```python
from build123d import *

# Parameters (mm, degrees)
F0_W     = 23
F0_H     = 95
F1_DEPTH = 9
F2_W     = 5
F2_H     = 95
F3_DEPTH = 5
F4_R     = 2
F5_DEPTH = 12.446


with BuildPart() as f1:
    # F0 (on Top) → F1 (new body)
    with BuildSketch(Plane.XY):
        Rectangle(F0_W, F0_H)
    extrude(amount=F1_DEPTH)

    # F2 (on face) → F3 (cut)
    with BuildSketch(Plane.XY.offset(9)):
        with Locations((-9, 0)):
            Rectangle(F2_W, F2_H)
    extrude(amount=-F3_DEPTH, mode=Mode.SUBTRACT)

    # F4 (on face) → F5 (cut)
    with BuildSketch(Plane.XY.offset(9)):
        with Locations((2.5, 35.605948)):
            Circle(F4_R)
        with Locations((2.5, -32.262102)):
            Circle(F4_R)
    extrude(amount=-F5_DEPTH, mode=Mode.SUBTRACT)


solid = f1.part
```
The listing builds one solid part. Answer for the finished solid, in the listing's coordinates (mm). A direction names the side the tool comes from. Give positions to 0.01 mm unless a question says otherwise; leave off trailing zeros. Loops run counter-clockwise (first coordinate to the right, second up) from the corner with the lowest first, then second, coordinate; pieces in that order, holes last. Notation, with made-up numbers: (4, 24.5) - (32, 24.5) arc R20 cw to (32, 53.5) - close; hole circle Ø11 at (-17, 9.25). An arc over 180 degrees is marked (long way). Return JSON: item names as keys, results as strings. Group by question number.
1. Find section B-B (z = 5.25). Write down the section's boundary in (x, y), then the cut area to 3 significant figures.
2. Given pin 1 Ø3.5 at (x, y) = (2.5, 35.61) entering from +Z; pin 2 Ø4 at (x, y) = (-9, -5) entering from +Z; pin 3 Ø5 at (y, z) = (-2, 7.5) entering from -X, each flat-ended and moving along its own axis, determine where each tip first touches the part or whether it passes through.
3. Determine the mould class of faces 1 (the cylindrical face through (2.24, -30.28, 4.56)), 2 (the flat face through (11.5, -1, 4)), 3 (the flat face through (-11.5, -1, 2)) for opening direction X: pulls with the +X half, pulls with the -X half, needs draft (parallel to the pull), parting line crosses it, or undercut.
4. Straight lines are drawn through the part: line 1 (Y direction, x = 2.5, z = 2.75); line 2 (Y direction, x = 1.25, z = 5.5); line 3 (X direction, y = -7, z = 7.75). For each, find the intervals that lie inside material, in ascending order. Write a range as [from, to].
5. Find section A-A (x = 2.5). Write down the section's boundary in (y, z).
6. Find section C-C (y = -18.5). Write down the section's boundary in (x, z), then the cut area to 3 significant figures.
7. Which of the six approach directions +Z, -Z, +X, -X, +Y, -Y give full straight-line access (tool end or side, diameter ignored) to faces 4 (the flat face through (0, 47.5, 4)), 5 (the flat face through (-9, 1, 4))?
Verdict:
{
 "1": {"outline": "(-6.5, -47.5) - (11.5, -47.5) - (11.5, 47.5) - (-6.5, 47.5) - close; hole circle Ø4 at (2.5, -32.26); hole circle Ø4 at (2.5, 35.61)", "area": "1,680 mm^2"},
 "2": {"pin 1": "passes through", "pin 2": "stops at z = 4", "pin 3": "stops at x = -6.5"},
 "3": {"face 1": "undercut", "face 2": "pulls with the +X half", "face 3": "pulls with the -X half"},
 "4": {"line 1": "y = [-47.5, -34.26], [-30.26, 33.61], [37.61, 47.5]", "line 2": "y = [-47.5, -33.82], [-30.7, 34.04], [37.17, 47.5]", "line 3": "x = [-6.5, 11.5]"},
 "5": {"outline": "(-47.5, 0) - (-34.26, 0) - (-34.26, 9) - (-47.5, 9) - close; (-30.26, 0) - (33.61, 0) - (33.61, 9) - (-30.26, 9) - close; (37.61, 0) - (47.5, 0) - (47.5, 9) - (37.61, 9) - close"},
 "6": {"outline": "(-11.5, 0) - (11.5, 0) - (11.5, 9) - (-6.5, 9) - (-6.5, 4) - (-11.5, 4) - close", "area": "182 mm^2"},
 "7": {"face 4": "+Z, -Z, +X, -X, +Y", "face 5": "+Z, -X, +Y, -Y"}
}
